Verification items for this drawing (mm, ordinates from the low corner). Coordinates: 2 decimals unless noted, no trailing zeros. Order: outer loops, then holes, each group sorted by start corner. A loop starts at its lowest first (then second) coordinate and runs counter-clockwise, first axis right, second up. Notation, with made-up numbers: M 55.25,69 L 90.25,69 A14 cw 90.25,88 Z; hole C 77.25,39.25 d10. An arc over 180 degrees is marked long. Return JSON: item names as keys, results as strings. Group by question number.
1. Section check B-B, the plane x = 12. Record the cut outline in (y, z), plus the area to 3 significant figures.
2. Gauge pin test, flat ends, axial feed: pin 1 (5 mm diameter, centred on y = 6, z = 21, fed in from +X); pin 2 (1 mm diameter, centred on y = 8.5, z = 18.5, fed in from -X); pin 3 (2 mm diameter, centred on y = 7, z = 9, fed in from +X). Record the tip position at first contact, or that the pin passes through.
3. Section check A-A, the plane z = 12. Record the cut outline in (x, y), plus the area to 3 significant figures.
4. Material ranges on line 1 along Z through (x, y) = (12, 7.4); line 2 along X through (y, z) = (8.4, 12), recorded low to high.
5. Section check C-C, the plane y = 4. Record the cut outline in (x, z).
6. Section check D-D, the plane y = 9.75. Record the cut outline in (x, z), plus the area to 3 significant figures.
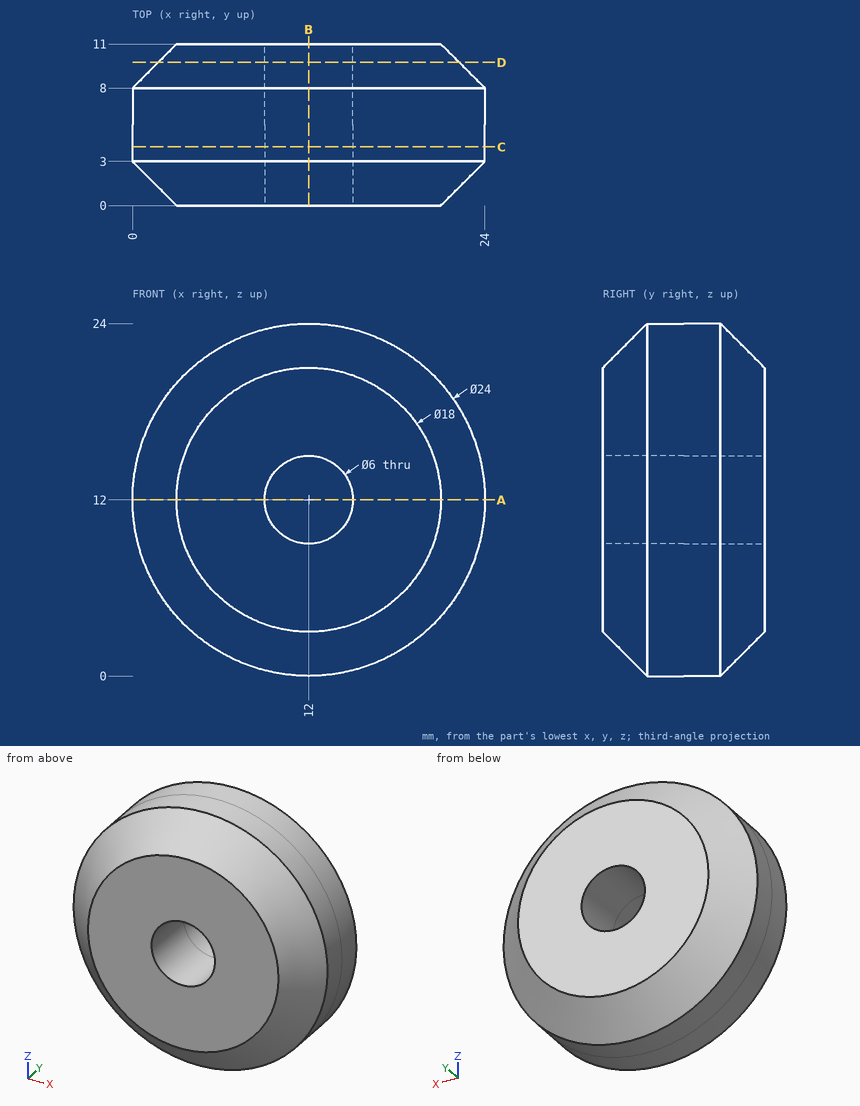
Answers follow:
{
 "1": {"outline": "M 0,3 L 3,0 L 8,0 L 11,3 L 11,9 L 0,9 Z; M 0,15 L 11,15 L 11,21 L 8,24 L 3,24 L 0,21 Z", "area": "180 mm^2"},
 "2": {"pin 1": "x = 22.09", "pin 2": "x = 1.83", "pin 3": "x = 23.83"},
 "3": {"outline": "M 0,3 L 3,0 L 9,0 L 9,11 L 3,11 L 0,8 Z; M 15,0 L 21,0 L 24,3 L 24,8 L 21,11 L 15,11 Z", "area": "180 mm^2"},
 "4": {"line 1": "0 to 9, 15 to 24", "line 2": "0.4 to 9, 15 to 23.6"},
 "5": {"outline": "C 12,12 d24; hole C 12,12 d6"},
 "6": {"outline": "C 12,12 d20.5; hole C 12,12 d6", "area": "302 mm^2"}
}
